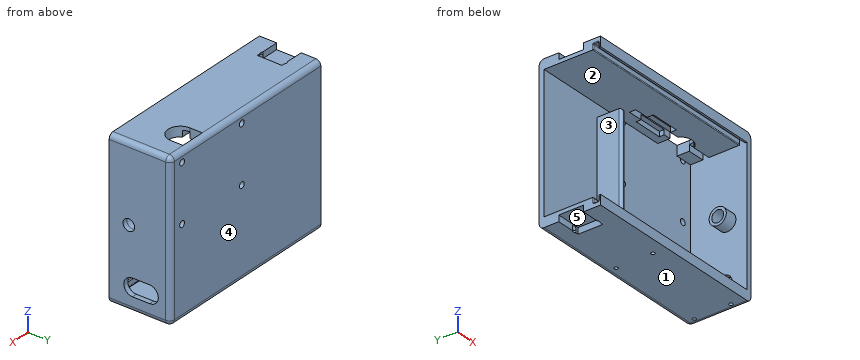
```python
from build123d import *

# Parameters (mm, degrees)
SKETCH1_W               = 80
SKETCH1_H               = 63
BOSS_EXTRUDE2_DEPTH     = 25
SKETCH1_4_W             = 76
SKETCH1_4_H             = 55
CUT_EXTRUDE1_DEPTH      = 23
SKETCH4_W               = 2
SKETCH4_H               = 55
BOSS_EXTRUDE3_DEPTH     = 10
FILLET1_R               = 2
SKETCH5_W               = 2
SKETCH5_H               = 63
CUT_EXTRUDE3_DEPTH      = 105.852277038
SKETCH6_W               = 2.2
SKETCH6_H               = 2.2
CUT_EXTRUDE4_DEPTH      = 76
SKETCH7_W               = 10
SKETCH7_H               = 10
CUT_EXTRUDE5_DEPTH      = 2.5
CUT_EXTRUDE6_DEPTH      = 11.5
CUT_EXTRUDE6_DEPTH_BACK = 1.5
SKETCH8_R               = 0.875
SKETCH9_W               = 10
SKETCH9_H               = 10
CUT_EXTRUDE7_DEPTH      = 2.5
CUT_EXTRUDE8_DEPTH      = 11.5
CUT_EXTRUDE8_DEPTH_BACK = 1.5
SKETCH10_R              = 0.875
CUT_EXTRUDE9_DEPTH      = 2
CUT_EXTRUDE10_DEPTH     = 2
FILLET2_R               = 0.3
CUT_EXTRUDE13_REACH     = 86.524
SKETCH15_W              = 5
SKETCH15_H              = 10
FILLET3_R               = 1
SKETCH18_R              = 2.35
CUT_EXTRUDE16_DEPTH     = 15
CUT_EXTRUDE16_DRAFT     = 2
SKETCH19_R              = 1.25
CUT_EXTRUDE17_DEPTH     = 10
CUT_EXTRUDE18_REACH     = 106.852
SKETCH17_R              = 5
SKETCH20_R              = 3.5
SKETCH20_R_2            = 2.419841539
BOSS_EXTRUDE4_DEPTH     = 5
SKETCH21_R              = 0.75
CUT_EXTRUDE19_DEPTH     = 10
SKETCH22_W              = 38
SKETCH22_H              = 2.5
CUT_EXTRUDE20_DEPTH     = 2.5
SKETCH23_W              = 10
SKETCH23_H              = 5
CUT_EXTRUDE21_DEPTH     = 10
SKETCH24_W              = 12
SKETCH24_H              = 7
CUT_EXTRUDE22_DEPTH     = 2
CUT_EXTRUDE23_DEPTH     = 2


with BuildPart() as part:
    # Sketch1 → Boss-Extrude2 (new body)
    with BuildSketch(Plane(origin=(0, 0, 0), x_dir=(1, 0, 0), z_dir=(0, 1, 0))):
        with Locations((40, 31.5)):
            Rectangle(SKETCH1_W, SKETCH1_H)
    extrude(amount=BOSS_EXTRUDE2_DEPTH)

    # Sketch1<4> → Cut-Extrude1 (cut)
    with BuildSketch(Plane(origin=(0, 0, 0), x_dir=(1, 0, 0), z_dir=(0, 1, 0))):
        with Locations((40, 31.5)):
            Rectangle(SKETCH1_4_W, SKETCH1_4_H)
    extrude(amount=CUT_EXTRUDE1_DEPTH, mode=Mode.SUBTRACT)

    # Sketch4 → Boss-Extrude3 (add)
    with BuildSketch(Plane.XZ.offset(-23)):
        with Locations((30.5, -31.5)):
            Rectangle(SKETCH4_W, SKETCH4_H)
    extrude(amount=BOSS_EXTRUDE3_DEPTH)

    # Fillet1
    fillet1_edges = [part.edges().sort_by_distance(p)[0] for p in [
        (80, 25, -31.5),
        (40, 25, 0),
        (0, 25, -31.5),
        (0, 12.5, 0),
        (80, 12.5, 0),
        (80, 12.5, -63),
        (0, 12.5, -63),
        (40, 25, -63),
    ]]
    fillet(fillet1_edges, radius=FILLET1_R)

    # Sketch5 → Cut-Extrude3 (cut, through all)
    with BuildSketch(Plane(origin=(0, 0, 0), x_dir=(-1, 0, 0), z_dir=(0, -1, 0))):
        with Locations((-1, 31.5)):
            Rectangle(SKETCH5_W, SKETCH5_H)
    extrude(amount=-CUT_EXTRUDE3_DEPTH, mode=Mode.SUBTRACT)

    # Sketch6 → Cut-Extrude4 (cut)
    with BuildSketch(Plane.ZY.offset(-2)):
        with Locations((-2.9, 1.85)):
            Rectangle(SKETCH6_W, SKETCH6_H)
        with Locations((-60.1, 1.85)):
            Rectangle(SKETCH6_W, SKETCH6_H)
    extrude(amount=-CUT_EXTRUDE4_DEPTH, mode=Mode.SUBTRACT)

    # Sketch7 → Cut-Extrude5 (cut)
    with BuildSketch(Plane(origin=(0, 0, -63), x_dir=(-1, 0, 0), z_dir=(0, 0, -1))):
        with Locations((-7, 12)):
            Rectangle(SKETCH7_W, SKETCH7_H)
    extrude(amount=-CUT_EXTRUDE5_DEPTH, mode=Mode.SUBTRACT)

    # Sketch8 → Cut-Extrude6 (cut, two sides: drawn at the far end of the back side and taken through both)
    with BuildSketch(Plane(origin=(0, 7, 0), x_dir=(1, 0, 0), z_dir=(0, 1, 0)).offset(-CUT_EXTRUDE6_DEPTH_BACK)):
        with Locations(Location((10, 61.5, 0), (0, 0, 270))):
            Circle(SKETCH8_R)
    extrude(amount=CUT_EXTRUDE6_DEPTH + CUT_EXTRUDE6_DEPTH_BACK, mode=Mode.SUBTRACT)

    # Sketch9 → Cut-Extrude7 (cut)
    with BuildSketch(Plane.XY):
        with Locations((7, 12)):
            Rectangle(SKETCH9_W, SKETCH9_H)
    extrude(amount=-CUT_EXTRUDE7_DEPTH, mode=Mode.SUBTRACT)

    # Sketch10 → Cut-Extrude8 (cut, two sides: drawn at the far end of the back side and taken through both)
    with BuildSketch(Plane(origin=(0, 7, 0), x_dir=(1, 0, 0), z_dir=(0, 1, 0)).offset(-CUT_EXTRUDE8_DEPTH_BACK)):
        with Locations((10, 1.5)):
            Circle(SKETCH10_R)
    extrude(amount=CUT_EXTRUDE8_DEPTH + CUT_EXTRUDE8_DEPTH_BACK, mode=Mode.SUBTRACT)

    # Sketch11 → Cut-Extrude9 (cut)
    with BuildSketch(Plane(origin=(0, 0, -63), x_dir=(-1, 0, 0), z_dir=(0, 0, -1))):
        with BuildLine():
            Line((-9.122986176, 7), (-10.8, 7))
            add(Edge.make_bspline(
                [(-10.8, 7), (-9.980201359, 6.395551325), (-9.122986176, 7)],
                knots=[0, 0, 0, 1, 1, 1], degree=2))
        make_face()
        with BuildLine():
            Line((-9.122986176, 17), (-10.8, 17))
            add(Edge.make_bspline(
                [(-10.8, 17), (-9.980201359, 17.604448675), (-9.122986176, 17)],
                knots=[0, 0, 0, 1, 1, 1], degree=2))
        make_face()
    extrude(amount=-CUT_EXTRUDE9_DEPTH, mode=Mode.SUBTRACT)

    # Sketch12 → Cut-Extrude10 (cut)
    with BuildSketch(Plane.XY):
        with BuildLine():
            Line((11, 7), (9.120131213, 7))
            add(Edge.make_bspline(
                [(11, 7), (10.05659536, 6.399803182), (9.120131213, 7)],
                knots=[0, 0, 0, 1, 1, 1], degree=2))
        make_face()
        with BuildLine():
            Line((11, 17), (9.120131213, 17))
            add(Edge.make_bspline(
                [(11, 17), (10.05659536, 17.600196818), (9.120131213, 17)],
                knots=[0, 0, 0, 1, 1, 1], degree=2))
        make_face()
    extrude(amount=-CUT_EXTRUDE10_DEPTH, mode=Mode.SUBTRACT)

    # Fillet2
    fillet2_edges = [part.edges().sort_by_distance(p)[0] for p in [
        (40, 2.95, -59),
        (2, 0.75, -60.1),
        (2, 1.85, -61.2),
        (40, 0.75, -61.2),
        (40, 2.95, -61.2),
        (2, 2.95, -60.1),
        (2, 2.95, -2.9),
        (40, 2.95, -4),
        (40, 2.95, -1.8),
        (40, 0.75, -1.8),
        (2, 0.75, -2.9),
        (2, 1.85, -1.8),
    ]]
    fillet(fillet2_edges, radius=FILLET2_R)

    # Sketch15 → Cut-Extrude13 (cut, up to next)
    with BuildSketch(Plane.ZY.offset(-29.5), mode=Mode.PRIVATE) as cut_extrude13_sk1:
        with Locations((-6.5, 18)):
            Rectangle(SKETCH15_W, SKETCH15_H)
    cut_extrude13_tool1 = extrude(cut_extrude13_sk1.sketch, amount=-CUT_EXTRUDE13_REACH, mode=Mode.PRIVATE) & part.part
    add(cut_extrude13_tool1.solids().sort_by_distance((29.5, 18, -6.5))[0], mode=Mode.SUBTRACT)

    # Fillet3
    fillet3_edges = [part.edges().sort_by_distance(p)[0] for p in [
        (29.5, 13, -34),
        (30.5, 13, -9),
        (29.5, 18, -59),
        (31.5, 18, -59),
        (30.5, 13, -59),
        (31.5, 13, -34),
    ]]
    fillet(fillet3_edges, radius=FILLET3_R - 0.0001)  # a hair under: the kernel refuses the full size


with BuildPart() as cut_extrude16_tool:
    # Sketch18 → Cut-Extrude16 (with draft: the straight prism first)
    with BuildSketch(Plane(origin=(80, 0, 0), x_dir=(0, 0, -1), z_dir=(1, 0, 0))):
        with Locations((31, 8)):
            Circle(SKETCH18_R)
    extrude(amount=-CUT_EXTRUDE16_DEPTH)
    # Cut-Extrude16: the draft: its side faces are tilted about the plane it starts from
    cut_extrude16_sides = [cut_extrude16_tool.faces().sort_by_distance(p)[0] for p in [
        (72.5, 8, -28.65),
    ]]
    draft(cut_extrude16_sides, Plane(origin=(80, 0, 0), x_dir=(0, 0, -1), z_dir=(1, 0, 0)), CUT_EXTRUDE16_DRAFT)


with BuildPart() as part_1:
    add(part.part)

    # Cut-Extrude16: cut by cut_extrude16_tool
    add(cut_extrude16_tool.part, mode=Mode.SUBTRACT)

    # Sketch19 → Cut-Extrude17 (cut)
    with BuildSketch(Plane.XZ.offset(-23)):
        with Locations(Location((74, -4.2, 0), (0, 0, 270))):
            Circle(SKETCH19_R)
        with Locations(Location((74, -27.2, 0), (0, 0, 270))):
            Circle(SKETCH19_R)
        with Locations(Location((43, -27.2, 0), (0, 0, 270))):
            Circle(SKETCH19_R)
        with Locations(Location((43, -4.2, 0), (0, 0, 270))):
            Circle(SKETCH19_R)
    extrude(amount=-CUT_EXTRUDE17_DEPTH, mode=Mode.SUBTRACT)

    # Sketch17 → Cut-Extrude18 (cut, up to next)
    with BuildSketch(Plane.XY, mode=Mode.PRIVATE) as cut_extrude18_sk1:
        with Locations(Location((66, 18, 0), (0, 0, 90))):
            Circle(SKETCH17_R)
    cut_extrude18_tool1 = extrude(cut_extrude18_sk1.sketch, amount=-CUT_EXTRUDE18_REACH, mode=Mode.PRIVATE) & part_1.part
    add(cut_extrude18_tool1.solids().sort_by_distance((66, 18, 0))[0], mode=Mode.SUBTRACT)

    # Sketch20 → Boss-Extrude4 (add)
    with BuildSketch(Plane.ZY.offset(-78)):
        with Locations((-31, 8)):
            Circle(SKETCH20_R)
        with Locations((-31, 8)):
            Circle(SKETCH20_R_2, mode=Mode.SUBTRACT)
    extrude(amount=BOSS_EXTRUDE4_DEPTH)

    # Sketch21 → Cut-Extrude19 (cut)
    with BuildSketch(Plane.XY.offset(-59)):
        with Locations((76.7, 20.5)):
            Circle(SKETCH21_R)
        with Locations((76.7, 5.5)):
            Circle(SKETCH21_R)
        with Locations((36.2, 5.5)):
            Circle(SKETCH21_R)
        with Locations((36.2, 20.5)):
            Circle(SKETCH21_R)
    extrude(amount=-CUT_EXTRUDE19_DEPTH, mode=Mode.SUBTRACT)

    # Sketch22 → Cut-Extrude20 (cut)
    with BuildSketch(Plane(origin=(0, 0, -4), x_dir=(-1, 0, 0), z_dir=(0, 0, -1))):
        with Locations((-59, 16.75)):
            Rectangle(SKETCH22_W, SKETCH22_H)
    extrude(amount=-CUT_EXTRUDE20_DEPTH, mode=Mode.SUBTRACT)

    # Sketch23 → Cut-Extrude21 (cut)
    with BuildSketch(Plane.XY):
        with Locations((66, 20.5)):
            Rectangle(SKETCH23_W, SKETCH23_H)
    extrude(amount=-CUT_EXTRUDE21_DEPTH, mode=Mode.SUBTRACT)

    # Sketch24 → Cut-Extrude22 (cut)
    with BuildSketch(Plane(origin=(0, 0, -4), x_dir=(-1, 0, 0), z_dir=(0, 0, -1))):
        with Locations((-52, 16.5)):
            Rectangle(SKETCH24_W, SKETCH24_H)
    extrude(amount=-CUT_EXTRUDE22_DEPTH, mode=Mode.SUBTRACT)

    # Sketch18<3> → Cut-Extrude23 (cut)
    with BuildSketch(Plane(origin=(80, 0, 0), x_dir=(0, 0, -1), z_dir=(1, 0, 0))):
        with BuildLine():
            Line((57.2, 16.5), (57.2, 9.5))
            ThreePointArc((57.2, 9.5), (53.7, 6), (50.2, 9.5))
            Line((50.2, 9.5), (50.2, 16.5))
            ThreePointArc((50.2, 16.5), (53.7, 20), (57.2, 16.5))
        make_face()
    extrude(amount=-CUT_EXTRUDE23_DEPTH, mode=Mode.SUBTRACT)


solid = part_1.part
```
Read the model definition and answer for the solid it produces. Units are mm, in the model's axes. Face numbers are marked on the shaded views. A direction names the side the tool comes from. Give positions to 0.01 mm unless a question says otherwise; leave off trailing zeros. Order: outer loops, then holes, each group sorted by start corner. A loop starts at its lowest first (then second) coordinate and runs counter-clockwise, first axis right, second up.
(1) Straight lines are drawn through the part: L1, parallel to Z at x = 75.5, y = 7.75; L2, parallel to Y at x = 76.7, z = -60.7; L3, parallel to X at y = 24.4, z = -4.2. For each, find the intervals that lie inside material, in ascending order.
(2) Given pin 1 (6 mm diameter, centred on y = 14, z = -37.5, fed in from -X); pin 2 (5 mm diameter, centred on x = 6.5, y = 10.5, fed in from -Z); pin 3 (4 mm diameter, centred on x = 11, z = -50.5, fed in from -Y), each flat-ended and moving along its own axis, determine where each tip first touches the part or whether it passes through.
(3) For the marked faces 1 and 2, determine the directions among +Z, -Z, +X, -X, +Y, -Y from which every point of the face is accessible in a straight line to the end or side of a thin tool.
(4) Find section D-D (y = 8). Give the vertices of the cut face in (x, z), plus the area to 3 significant figures.
(5) For a pull along Y with two mould halves and no side action, classify the marked faces 3, 4 and 5 as released by +Y, released by -Y, zero draft, split by the parting line, or undercut.
(6) Find section B-B (x = 66). Give the vertices of the cut face in (y, z).
Result sheet:
1. L1: z = -63 to -59, -34.49 to -33.41, -28.59 to -27.51, -4 to 0
1. L2: y = 0 to 0.75, 2.95 to 4.75, 6.25 to 19.75, 21.25 to 25
1. L3: x = 2 to 41.75, 44.25 to 72.75, 75.25 to 79.43
2. pin 1: stops at x = 29.5
2. pin 2: stops at z = -60.5
2. pin 3: stops at y = 23
3. face 1: -Z, +X, -X, +Y, -Y
3. face 2: -X, -Y
4. outline: (2, -60.5) - (12, -60.5) - (12, -63) - (78, -63) arc R2 ccw to (80, -61) - (80, -56.86) - (78, -56.86) - (78, -59) - (2, -59) - close; (2, -4) - (78, -4) - (78, -27.5) - (73, -27.5) - (73, -28.58) - (78, -28.58) - (80, -28.65) - (80, -2) arc R2 ccw to (78, 0) - (12, 0) - (12, -2.5) - (2, -2.5) - close; (73, -34.5) - (78, -34.5) - (78, -50.54) - (80, -50.54) - (80, -33.35) - (78, -33.42) - (73, -33.42) - close
4. area: 671 mm2
5. face 3: zero draft
5. face 4: released by +Y
5. face 5: undercut
6. outline: (0, -63) - (23, -63) arc R2 ccw to (25, -61) - (25, -2) arc R2 ccw to (23, 0) - (23, -59) - (3.25, -59) arc R0.3 ccw to (2.95, -59.3) - (2.95, -60.9) arc R0.3 cw to (2.65, -61.2) - (1.05, -61.2) arc R0.3 cw to (0.75, -60.9) - (0.75, -59) - (0, -59) - close; (0, -4) - (0.75, -4) - (0.75, -2.1) arc R0.3 cw to (1.05, -1.8) - (2.65, -1.8) arc R0.3 cw to (2.95, -2.1) - (2.95, -3.7) arc R0.3 ccw to (3.25, -4) - (13, -4) - (13, 0) - (0, 0) - close
